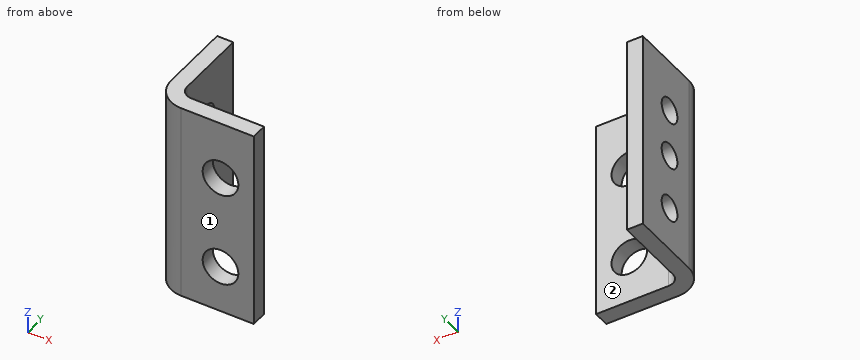
```python
from build123d import *

# Parameters (mm, degrees)
SKETCH1_W                    = 12.7
SKETCH1_H                    = 6.35
SKETCH1_R                    = 0.785
BASE_FLANGE1_DEPTH           = 1.016
EDGE_FLANGE1_STRIP_W         = 5.5372
EDGE_FLANGE1_STRIP_H         = 1.016
EDGE_FLANGE1_STRIP_CUT_DEPTH = 12.7
EDGE_FLANGE1_DEPTH           = 12.7
CUT_EXTRUDE1_REACH           = 16.771
SKETCH9_R                    = 1.13


# Sheet-metal steps are written as plain solids
with BuildPart() as part:
    # Sketch1 → Base-Flange1 (new body)
    with BuildSketch(Plane(origin=(0, 0, 0), x_dir=(0, 0, -1), z_dir=(1, 0, 0))):
        with Locations((6.35, 3.175)):
            Rectangle(SKETCH1_W, SKETCH1_H)
        with Locations((3.3, 3.685)):
            Circle(SKETCH1_R, mode=Mode.SUBTRACT)
        with Locations((6.35, 3.685)):
            Circle(SKETCH1_R, mode=Mode.SUBTRACT)
        with Locations((9.91, 3.685)):
            Circle(SKETCH1_R, mode=Mode.SUBTRACT)
    extrude(amount=-BASE_FLANGE1_DEPTH)

    # Edge-Flange1 strip (across the edge) → Edge-Flange1 strip cut (cut)
    with BuildSketch(Plane.YX):
        with Locations((-1.016, -0.508)):
            Rectangle(EDGE_FLANGE1_STRIP_W, EDGE_FLANGE1_STRIP_H)
    extrude(amount=EDGE_FLANGE1_STRIP_CUT_DEPTH, mode=Mode.SUBTRACT)

    # Edge-Flange1 section (across the edge) → Edge-Flange1 (add)
    with BuildSketch(Plane.YX):
        with BuildLine():
            Line((0, 0.7366), (0, 5.334))
            Line((0, 5.334), (1.016, 5.334))
            Line((1.016, 5.334), (1.016, 0.7366))
            ThreePointArc((1.016, 0.7366), (1.231745145, 0.215745145), (1.7526, 0))
            Line((1.7526, 0), (1.7526, -1.016))
            ThreePointArc((1.7526, -1.016), (0.513324655, -0.502675345), (0, 0.7366))
        make_face()
    extrude(amount=EDGE_FLANGE1_DEPTH)

    # Sketch9 → Cut-Extrude1 (cut, up to next)
    with BuildSketch(Plane(origin=(0, 1.016, 0), x_dir=(1, 0, 0), z_dir=(0, 1, 0)), mode=Mode.PRIVATE) as cut_extrude1_sk1:
        with Locations(Location((3.224, 3.7, 0), (0, 0, 180))):
            Circle(SKETCH9_R)
    cut_extrude1_tool1 = extrude(cut_extrude1_sk1.sketch, amount=-CUT_EXTRUDE1_REACH, mode=Mode.PRIVATE) & part.part
    # Sketch9 → Cut-Extrude1 (cut, up to next)
    with BuildSketch(Plane(origin=(0, 1.016, 0), x_dir=(1, 0, 0), z_dir=(0, 1, 0)), mode=Mode.PRIVATE) as cut_extrude1_sk2:
        with Locations(Location((3.224, 9.7, 0), (0, 0, 180))):
            Circle(SKETCH9_R)
    cut_extrude1_tool2 = extrude(cut_extrude1_sk2.sketch, amount=-CUT_EXTRUDE1_REACH, mode=Mode.PRIVATE) & part.part
    add(cut_extrude1_tool1.solids().sort_by_distance((3.224, 1.016, -3.7))[0], mode=Mode.SUBTRACT)
    add(cut_extrude1_tool2.solids().sort_by_distance((3.224, 1.016, -9.7))[0], mode=Mode.SUBTRACT)


solid = part.part
```
Work out the finished part from the listing and answer in its coordinate system (mm). Face numbers are marked on the shaded views. A direction names the side the tool comes from. Give positions to 0.01 mm unless a question says otherwise; leave off trailing zeros. Order: outer loops, then holes, each group sorted by start corner. A loop starts at its lowest first (then second) coordinate and runs counter-clockwise, first axis right, second up.
1. For the marked faces 1 and 2, determine the directions among +Z, -Z, +X, -X, +Y, -Y from which every point of the face is accessible in a straight line to the end or side of a thin tool.
Result sheet:
face 1: +Z, -Z, +X, -X, -Y
face 2: +Z, -Z, +X, +Y
2. Each of these flat-tipped pins is pushed along its axis until it touches: P1, Ø2, axis at y = 2.5, z = -7, coming from the +X side; P2, Ø2.5, axis at x = 3.5, z = -3.5, coming from the +Y side; P3, Ø1.4, axis at y = 3.685, z = -3.3, coming from the +X side. Where does it stop, or does it pass through?
Result sheet:
P1: stops at x = 0.04
P2: stops at y = 1.02
P3: passes through
3. Section D-D, the plane z = -9 is taken. Determine the outline of the cut face in (x, y), and give its area (3 significant figures).
Result sheet:
outline: (-1.02, 1.75) arc R1.75 ccw to (0.74, 0) - (2.34, 0) - (2.34, 1.02) - (0.74, 1.02) arc R0.74 cw to (0, 1.75) - (0, 6.35) - (-1.02, 6.35) - close; (4.11, 0) - (5.33, 0) - (5.33, 1.02) - (4.11, 1.02) - close
area: 9.53 mm2
4. Section C-C, the plane z = -3.7 is taken. Determine the outline of the cut face in (x, y), and give its area (3 significant figures).
Result sheet:
outline: (-1.02, 1.75) arc R1.75 ccw to (0.74, 0) - (2.09, 0) - (2.09, 1.02) - (0.74, 1.02) arc R0.74 cw to (0, 1.75) - (0, 3.01) - (-1.02, 3.01) - close; (-1.02, 4.36) - (0, 4.36) - (0, 6.35) - (-1.02, 6.35) - close; (4.35, 0) - (5.33, 0) - (5.33, 1.02) - (4.35, 1.02) - close
area: 7.66 mm2
5. Section B-B, the plane x = 4 is taken. Determine the outline of the cut face in (y, z).
Result sheet:
outline: (0, -12.7) - (1.02, -12.7) - (1.02, -10.52) - (0, -10.52) - close; (0, -8.88) - (1.02, -8.88) - (1.02, -4.52) - (0, -4.52) - close; (0, -2.88) - (1.02, -2.88) - (1.02, 0) - (0, 0) - close
6. Straight lines are drawn through the part: L1, parallel to Z at x = 2.25, y = 0.75; L2, parallel to X at y = 4.5, z = -3; L3, parallel to Y at x = -0.3, z = -9.91. For each, find the intervals that lie inside material, in ascending order.
Result sheet:
L1: z = -12.7 to -10.27, -9.13 to -4.27, -3.13 to 0
L2: x = -1.02 to 0
L3: y = 0.34 to 2.9, 4.47 to 6.35
7. Section A-A, the plane z = -5.25 is taken. Determine the outline of the cut face in (x, y), and give its area (3 significant figures).
Result sheet:
outline: (-1.02, 1.75) arc R1.75 ccw to (0.74, 0) - (5.33, 0) - (5.33, 1.02) - (0.74, 1.02) arc R0.74 cw to (0, 1.75) - (0, 6.35) - (-1.02, 6.35) - close
area: 11.3 mm2
